Input: part model. Units: mm. Frame: model coordinates. Face numbers are marked on the shaded views. A direction names the side the tool comes from. Round coordinates to 2 decimals unless told otherwise and drop trailing zeros. Loops run counter-clockwise (first coordinate to the right, second up) from the corner with the lowest first, then second, coordinate; pieces in that order, holes last. Notation, with made-up numbers: M 66,21 L 88,21 A23 cw 88,56 Z; hole C 24.25,51 d4. An arc over 180 degrees is marked long. Put each result on its own line as item: value. Start each with the question number.
1) Pin query (flat end, axial travel): pin 1 (4 mm diameter, centred on x = -40.5, z = -71, fed in from -Y). Return the tip coordinate at first contact, or that it passes through.
2) Line query: probe 1 along Z at (x, y) = (-80.5, -75); probe 2 along Y at (x, z) = (-97, 39); probe 3 along X at (y, z) = (4.5, -176). Output: solid intervals per line, ascending.
3) Section B-B on z = 23. Output: boundary loops of the cut face in (x, y).
4) Reachability of the marked faces 1, 2, 3, 4 and 5 from +Z, -Z, +X, -X, +Y, -Y: full face, straight path, thin tool, end or side. Return the list, or none.
5) Draft query along Y for the marked faces 6, 7 and 8. Return one class per face: +Y half, -Y half, draft (parallel to the pull), parting line (faces both ways), or undercut.
6) Section C-C on x = -50.5. Output: boundary loops of the cut face in (y, z), plus the area to 3 significant figures.
7) Section D-D on z = -181.5. Output: boundary loops of the cut face in (x, y).
Autodesk Inventor part; units mm, degrees
ref_plane "YZ Plane" through (0, 0, 0) normal (1, 0, 0) x (0, 1, 0)
ref_plane "XZ Plane" through (0, 0, 0) normal (0, 1, 0) x (-1, 0, 0)
ref_plane "XY Plane" through (0, 0, 0) normal (0, 0, 1) x (1, 0, 0)
sketch "Sketch1" plane through (0, 0, 0) normal (0, 0, 1) x (1, 0, 0)
  line L0 (-101.6, 50.8) -> (0, 50.8)
  line L1 (0, 50.8) -> (0, 0)
  line L2 (0, 0) -> (-101.6, 0)
  line L3 (-101.6, 0) -> (-101.6, 50.8)
  dimension "d0" = 101.6
  dimension "d1" = 50.8
extrude "Extrusion1" add sketch "Sketch1" along normal blind 76.2
sketch "Sketch2" plane through (-101.6, 0, 0) normal (0, -1, 0) x (1, 0, 0)
  line L0 (0, 0) -> (0, 76.2)
  line L1 (101.6, 0) -> (0, 0)
  line L2 (0, 0) -> (0, 9.5563)
  line L3 (0, 9.5563) -> (101.6, 9.5563)
  line L4 (101.6, 9.5563) -> (101.6, 0)
extrude "Extrusion2" add sketch "Sketch2" along normal blind 50.8
sketch "Sketch3" plane through (0, 0, 0) normal (0, 0, -1) x (-1, 0, 0)
  line L0 (101.6, -50.8) -> (0, -50.8)
  line L1 (0, -50.8) -> (0, -101.6194)
  line L2 (0, -101.6194) -> (101.6, -101.6194)
  line L3 (101.6, -101.6194) -> (101.6, -50.8)
  point P0 (0, 0)
extrude "Extrusion3" add sketch "Sketch3" against normal blind 76.2
sketch "Sketch4" plane through (0, 0, 0) normal (0, 0, -1) x (-1, 0, 0)
  line L0 (0, -101.6194) -> (0, 50.8)
  line L1 (101.6, 50.8) -> (101.6, -101.6194)
  line L2 (101.6, 0) -> (0, 0)
  line L3 (0, 0) -> (0, -50.8671)
  line L4 (0, -50.8671) -> (101.6, -50.8671)
  line L5 (101.6, -50.8671) -> (101.6, 0)
  point P0 (0, 0)
extrude "Extrusion4" add sketch "Sketch4" along normal blind 152.4
sketch "Sketch5" plane through (0, 0, -152.4) normal (0, 0, -1) x (-1, 0, 0)
  line L0 (0, -76.278) -> (101.6, -76.278)
  line L1 (101.6, -76.278) -> (101.6, 25.322)
  line L2 (101.6, 25.322) -> (0, 25.322)
  line L3 (0, 25.322) -> (0, -76.278)
  dimension "d10" = 101.6
  dimension "d11" = 101.6
extrude "Extrusion5" add sketch "Sketch5" along normal blind 101.6
sketch "Sketch6" plane through (-101.6, 25.322, -152.4) normal (0, 1, 0) x (1, 0, 0)
  line L0 (0, 0) -> (101.6, 0)
  line L1 (12.7038, 76.4129) -> (38.1038, 76.4129)
  line L2 (38.1038, 76.4129) -> (38.1038, 51.0129)
  line L3 (38.1038, 51.0129) -> (12.7038, 51.0129)
  line L4 (12.7038, 51.0129) -> (12.7038, 76.4129)
  line L5 (63.1592, 76.7092) -> (88.5592, 76.7092)
  line L6 (88.5592, 76.7092) -> (88.5592, 51.3092)
  line L7 (88.5592, 51.3092) -> (63.1592, 51.3092)
  line L8 (63.1592, 51.3092) -> (63.1592, 76.7092)
  line L9 (37.1295, 0) -> (29.2048, 0)
  point P0 (101.6, -152.4)
  dimension "d14" = 25.4
  dimension "d15" = 25.4
  dimension "d16" = 25.4
  dimension "d17" = 25.4
extrude "Extrusion6" cut sketch "Sketch6" against normal blind 25.4
sketch "Sketch7" plane through (-101.6, 25.322, -152.4) normal (0, 1, 0) x (1, 0, 0)
  line L0 (25.3513, 38.6799) -> (38.4727, 38.6799)
  line L1 (38.4727, 38.6799) -> (38.4727, 0.5799)
  line L2 (38.4727, 0.5799) -> (25.3513, 0.5799)
  line L3 (25.3513, 0.5799) -> (25.3513, 38.6799)
  line L4 (64.117, 38.5479) -> (76.0531, 38.5479)
  line L5 (76.0531, 38.5479) -> (76.0531, 0.4479)
  line L6 (76.0531, 0.4479) -> (64.117, 0.4479)
  line L7 (64.117, 0.4479) -> (64.117, 38.5479)
  point P0 (101.6, -152.4)
  dimension "d20" = 38.1
  dimension "d21" = 38.1
extrude "Extrusion7" cut sketch "Sketch7" against normal blind 25.4
sketch "Sketch8" plane through (-101.6, 25.322, -152.4) normal (0, 1, 0) x (1, 0, 0)
  line L0 (76.0531, 38.5479) -> (76.0531, 0.4479)
  line L1 (25.3513, 38.6799) -> (76.0531, 38.6799)
  line L2 (76.0531, 38.6799) -> (76.0531, 13.2799)
  line L3 (76.0531, 13.2799) -> (25.3513, 13.2799)
  line L4 (25.3513, 13.2799) -> (25.3513, 38.6799)
  point P0 (101.6, -152.4)
  dimension "d24" = 25.4
extrude "Extrusion8" cut sketch "Sketch8" against normal blind 25.4
sketch "Sketch9" plane through (-76.2487, 25.322, -152.9799) normal (1, 0, 0) x (0, 0, -1)
  line L0 (0, 0) -> (38.1, 0)
  line L1 (0, 0) -> (0, -25.4)
  line L2 (38.1, -25.4) -> (0, -25.4)
  line L3 (38.1, 0) -> (38.1, -25.4)
  point P0 (-152.9799, -25.322)
sketch "Sketch10" plane through (-101.6, 25.322, -152.4) normal (0, 1, 0) x (1, 0, 0)
  line L0 (25.3513, 38.6799) -> (76.0531, 38.6799)
  line L1 (38.1038, 51.0129) -> (63.1592, 51.0129)
  line L2 (63.1592, 51.0129) -> (63.1592, 38.6799)
  line L3 (63.1592, 38.6799) -> (38.1038, 38.6799)
  line L4 (38.1038, 38.6799) -> (38.1038, 51.0129)
  point P0 (101.6, -152.4)
extrude "Extrusion9" cut sketch "Sketch10" against normal blind 25.4
sketch "Sketch11" plane through (-101.6, -0.078, -152.4) normal (0, 1, 0) x (1, 0, 0)
  line L0 (88.5592, 76.7092) -> (75.8592, 76.7092)
  line L1 (75.8592, 76.7092) -> (75.8592, 64.0092)
  line L2 (75.8592, 64.0092) -> (88.5592, 64.0092)
  line L3 (88.5592, 64.0092) -> (88.5592, 76.7092)
  point P0 (101.6, -152.4)
extrude "Extrusion10" add sketch "Sketch11" along normal blind 12.7
sketch "Sketch12" plane through (-101.6, -0.078, -152.4) normal (0, 1, 0) x (1, 0, 0)
  line L0 (12.7038, 76.4129) -> (25.4038, 76.4129)
  line L1 (25.4038, 76.4129) -> (25.4038, 63.4415)
  line L2 (25.4038, 63.4415) -> (12.7038, 63.4415)
  line L3 (12.7038, 63.4415) -> (12.7038, 76.4129)
  point P0 (101.6, -152.4)
extrude "Extrusion11" add sketch "Sketch12" along normal blind 12.7
sketch "Sketch13" plane through (-63.1273, 25.322, -152.9799) normal (0, 0, -1) x (-1, 0, 0)
  line L0 (13.1215, -25.4) -> (0, -25.4)
  line L1 (13.1215, 0) -> (13.1215, -25.4)
  line L2 (0, 0) -> (13.1215, 0)
  line L3 (0, 0) -> (0, -25.4)
  point P0 (-63.1273, -25.322)
extrude "Extrusion12" add sketch "Sketch13" along normal blind 5.08
sketch "Sketch14" plane through (-25.5469, 25.322, -152.8479) normal (0, 0, -1) x (-1, 0, 0)
  line L0 (11.9361, -25.4) -> (0, -25.4)
  line L1 (11.9361, 0) -> (11.9361, -25.4)
  line L2 (0, 0) -> (11.9361, 0)
  line L3 (0, 0) -> (0, -25.4)
  point P0 (-25.5469, -25.322)
extrude "Extrusion13" add sketch "Sketch14" along normal blind 5.08
properties part number "Creeper"
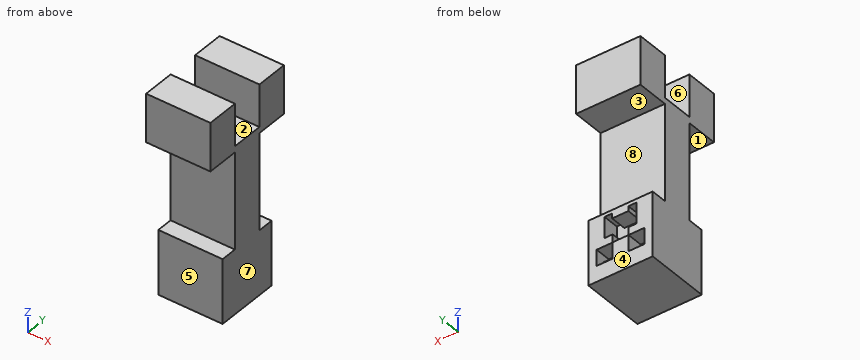
Geometry results:
1. pin 1: stops at y = -50.87
2. probe 1: z = -254 to -152.4, 0 to 76.2
2. probe 2: y = -101.62 to -50.8, 0 to 50.8
2. probe 3: x = -101.6 to -76.25, -25.55 to 0
3. outline: M -101.6,-101.62 L 0,-101.62 L 0,-50.8 L -101.6,-50.8 Z; M -101.6,0 L 0,0 L 0,50.8 L -101.6,50.8 Z
4. face 1: +X, -X, -Y
4. face 2: +Z, +X, -X
4. face 3: +X, -X, +Y
4. face 4: -Z, +X, -X, +Y
4. face 5: -Z, +X, -X, -Y
5. face 6: undercut
5. face 7: draft
5. face 8: +Y half
6. outline: M -101.62,0 L -50.87,0 L -50.87,-152.4 L -76.28,-152.4 L -76.28,-254 L 25.32,-254 L 25.32,-203.41 L -0.08,-203.41 L -0.08,-165.68 L 25.32,-165.68 L 25.32,-152.4 L 0,-152.4 L 0,0 L 50.8,0 L 50.8,76.2 L 0,76.2 L 0,9.56 L -50.8,9.56 L -50.8,76.2 L -101.62,76.2 Z
6. area: 25,300 mm²
7. outline: M -101.6,-76.28 L 0,-76.28 L 0,25.32 L -25.55,25.32 L -25.55,-0.08 L -76.25,-0.08 L -76.25,25.32 L -101.6,25.32 Z
